from build123d import *

# Parameters (mm, degrees)
SKETCH003_R          = 30
PAD001_DEPTH         = 5
SKETCH004_R          = 2
PAD002_DEPTH         = 6
SKETCH005_R          = 3
POCKET002_DEPTH      = 5.001
POCKET002_DEPTH_BACK = 6.001
CHAMFER002_SIZE      = 1


with BuildPart() as part:
    # Sketch003 → Pad001 (new body)
    with BuildSketch(Plane.XY):
        Circle(SKETCH003_R)
    extrude(amount=PAD001_DEPTH)

    # Sketch004 (on Face3 of Pad001) → Pad002 (join)
    with BuildSketch(Plane.XY.offset(5)):
        with Locations((0, 23.0943)):
            Circle(SKETCH004_R)
        with BuildLine():
            ThreePointArc((-15.422876, 9.280888), (0, -18), (15.422876, 9.280888))
            ThreePointArc((-15.422876, 9.280888), (0, 6.188), (15.422876, 9.280888))
        make_face()
    extrude(amount=PAD002_DEPTH)

    # Sketch005 (on Face3 of Pad002) → Pocket002 (cut, two sides)
    with BuildSketch(Plane.XY.offset(5)) as pocket002_sk:
        Circle(SKETCH005_R)
    extrude(amount=-POCKET002_DEPTH, mode=Mode.SUBTRACT)
    extrude(pocket002_sk.sketch, amount=POCKET002_DEPTH_BACK, mode=Mode.SUBTRACT)

    # Chamfer002
    chamfer002_edges = [part.edges().sort_by_distance(p)[0] for p in [
        (30, 0, 2.5),
        (-30, 0, 0),
        (-30, 0, 5),
        (-3, 0, 0),
        (0, -18, 5),
        (0, 6.188, 5),
        (-2, 23.0943, 5),
        (-3, 0, 11),
        (3, 0, 5.5),
        (-15.422876, 9.280888, 8),
        (15.422876, 9.280888, 8),
        (0, -18, 11),
        (0, 6.188, 11),
        (2, 23.0943, 8),
        (-2, 23.0943, 11),
    ]]
    chamfer(chamfer002_edges, length=CHAMFER002_SIZE)


solid = part.part
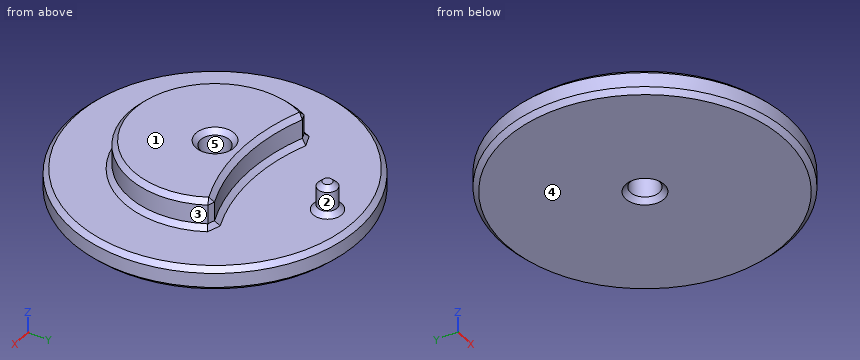
The listing builds one solid part. Answer for the finished solid, in the listing's coordinates (mm). Face numbers are marked on the shaded views. A direction names the side the tool comes from. Give positions to 0.01 mm unless a question says otherwise; leave off trailing zeros. Write each loop counter-clockwise with the first axis right and the second up, starting at its lowest first coordinate (ties: lowest second). Pieces come first, ordered by that corner, then holes. Notation, with made-up numbers: (10.25, 80.25) - (38.25, 80.25) arc R16 cw to (38.25, 91.25) - close; hole circle Ø9 at (74, 82). An arc over 180 degrees is marked (long way). Use a Markdown table: item, result.
1. For a pull along Y with two mould halves and no side action, classify the marked faces 3, 4 and 5 as released by +Y, released by -Y, zero draft, split by the parting line, or undercut.
Values follow:
| item | result |
|---|---|
| face 3 | split by the parting line |
| face 4 | zero draft |
| face 5 | undercut |
2. Section D-D on z = 7.25 is taken. Count the separate pieces of the cut face and the enclosed holes in it, plus the area to 3 significant figures.
Values follow:
| item | result |
|---|---|
| separate pieces | 2 |
| enclosed holes | 1 |
| area | 747 mm² |
3. Find the intervals of material crossed by probe 1 along X at (y, z) = (0, 8); probe 2 along Y at (x, z) = (0, 5.5); probe 3 along Y at (x, z) = (0, 5.75), in increasing order. Write a range as from..to.
Values follow:
| item | result |
|---|---|
| probe 1 | x = -18..-3, 3..18 |
| probe 2 | y = -18.5..-3, 3..6.69, 20.59..25.59 |
| probe 3 | y = -18.25..-3, 3..6.44, 20.84..25.34 |
4. Each of these flat-tipped pins is pushed along its axis until it touches: P1, Ø12, axis at x = 17, y = -14.5, coming from the -Z side; P2, Ø2, axis at x = -7, y = 16.5, coming from the +Z side; P3, Ø4, axis at x = -16, z = 2, coming from the +Y side; P4, Ø3, axis at x = 18.5, z = 2.5, coming from the +Y side. Where does it stop, or does it pass through?
Values follow:
| item | result |
|---|---|
| P1 | stops at z = 0 |
| P2 | stops at z = 5 |
| P3 | stops at y = 26.53 |
| P4 | stops at y = 24.72 |
5. Section A-A on y = 0 is taken. Write down the section's boundary in (x, z), plus the area to 3 significant figures.
Values follow:
| item | result |
|---|---|
| outline | (-30, 1) - (-29, 0) - (-4, 0) - (-3, 1) - (-3, 10) - (-4, 11) - (-17, 11) - (-18, 10) - (-18, 6) - (-19, 5) - (-29, 5) - (-30, 4) - close; (3, 1) - (4, 0) - (29, 0) - (30, 1) - (30, 4) - (29, 5) - (19, 5) - (18, 6) - (18, 10) - (17, 11) - (4, 11) - (3, 10) - close |
| area | 446 mm² |
6. A tool of negligible diameter and unlimited length cuts with its end or side. For the marked faces 1 and 2, from which of +Z, -Z, +X, -X, +Y, -Y can it reach the whole face along a straight path? Write none if from no direction.
Values follow:
| item | result |
|---|---|
| face 1 | +Z, +X, -X, +Y, -Y |
| face 2 | +Z |
7. Section B-B on z = 2.75 is taken. Write down the section's boundary in (x, y), plus the area to 3 significant figures.
Values follow:
| item | result |
|---|---|
| outline | circle Ø60 at (0, 0); hole circle Ø6 at (0, 0) |
| area | 2,800 mm² |
